Autodesk Inventor part; units mm, degrees
ref_plane "YZ Plane" through (0, 0, 0) normal (1, 0, 0) x (0, 1, 0)
ref_plane "XZ Plane" through (0, 0, 0) normal (0, 1, 0) x (-1, 0, 0)
ref_plane "XY Plane" through (0, 0, 0) normal (0, 0, 1) x (1, 0, 0)
sketch "Sketch1" plane through (0, 0, 0) normal (1, 0, 0) x (0, 1, 0)
  line L0 (0, 0) -> (103.378, 0)
  line L1 (103.378, 0) -> (103.378, -444.5)
  line L2 (103.378, -444.5) -> (0, -444.5)
  line L3 (0, -444.5) -> (0, 0)
  circle A0 centre (31.75, -50.8) radius 6.3627
  circle A1 centre (31.75, -393.7) radius 6.3627
  circle A2 centre (88.0618, -165.5318) radius 1.5875
  circle A3 centre (72.0598, -165.5318) radius 1.5875
  circle A4 centre (15.3162, -278.9682) radius 1.5875
  circle A5 centre (31.3182, -278.9682) radius 1.5875
  dimension "d0" = 103.378
  dimension "d1" = 444.5
  dimension "d2" = 12.7254
  dimension "d3" = 31.75
  dimension "d4" = 50.8
  dimension "d5" = 50.8
  dimension "d22" = 165.5318
  dimension "d23" = 3.175
  dimension "d24" = 15.3162
  dimension "d25" = 3.175
  dimension "d26" = 16.002
  dimension "d27" = 165.5318
  dimension "d28" = 3.175
  dimension "d29" = 15.3162
  dimension "d30" = 165.5318
  dimension "d31" = 3.175
  dimension "d32" = 16.002
  dimension "d33" = 165.5318
extrude "Extrusion1" add sketch "Sketch1" along normal blind 6.35 contours L0 L1 L2 L3 | A2 | A3 | A4 | A5
chamfer "Chamfer1" distance 38.1 angle 45 1 edges at (3.175, 0, 0)
chamfer "Chamfer2" distance 38.1 angle 45 1 edges at (3.175, 0, -444.5)
sketch "Sketch2" plane through (6.35, 0, 0) normal (1, 0, 0) x (0, 0, -1)
  line L0 (444.5, 38.1) -> (406.4, 0)
  line L1 (444.5, 38.1) -> (444.5, 103.378)
  line L2 (444.5, 103.378) -> (0, 103.378)
  line L3 (0, 103.378) -> (0, 38.1)
  line L4 (38.1, 0) -> (0, 38.1)
  line L5 (38.1, 0) -> (406.4, 0)
  circle A0 centre (393.7, 31.75) radius 6.3627
  circle A1 centre (50.8, 31.75) radius 6.3627
  circle A2 centre (120.4214, 66.0654) radius 6.3627
  circle A3 centre (324.0786, 37.3126) radius 6.3627
  point P0 (0, 0)
  dimension "d14" = 12.7254
  dimension "d15" = 120.4214
  dimension "d16" = 37.3126
  dimension "d17" = 12.7254
  dimension "d18" = 37.3126
  dimension "d19" = 120.4214
extrude "Extrusion2" cut sketch "Sketch2" against normal blind 25.4 contours A2 | A3
sketch "Sketch3" plane through (6.35, 0, 0) normal (1, 0, 0) x (0, 0, -1)
  circle A0 centre (120.4214, 66.0654) radius 6.3627
  circle A1 centre (324.0786, 37.3126) radius 6.3627
  line L0 (444.5, 38.1) -> (406.4, 0)
  line L1 (444.5, 38.1) -> (444.5, 103.378)
  line L2 (444.5, 103.378) -> (0, 103.378)
  line L3 (0, 103.378) -> (0, 38.1)
  line L4 (38.1, 0) -> (0, 38.1)
  line L5 (38.1, 0) -> (406.4, 0)
  circle A2 centre (393.7, 31.75) radius 6.3627
  circle A3 centre (50.8, 31.75) radius 6.3627
  circle A4 centre (165.5318, 88.0618) radius 1.5875
  circle A5 centre (165.5318, 72.0598) radius 1.5875
  circle A6 centre (278.9682, 15.3162) radius 1.5875
  circle A7 centre (278.9682, 31.3182) radius 1.5875
  point P0 (0, 0)
  dimension "d34" = 3.175
  dimension "d35" = 165.5318
  dimension "d36" = 15.3162
  dimension "d37" = 3.175
  dimension "d38" = 16.002
  dimension "d39" = 3.175
  dimension "d40" = 3.175
  dimension "d41" = 15.3162
  dimension "d42" = 16.002
  dimension "d43" = 165.5318
extrude "Extrusion3" cut sketch "Sketch3" against normal blind 25.4 contours A4 | A5 | A6 | A7
sketch "Sketch4" plane through (6.35, 0, 0) normal (1, 0, 0) x (0, 0, -1)
  circle A0 centre (278.9682, 15.3162) radius 1.5875
  circle A1 centre (165.5318, 88.0618) radius 1.5875
  circle A2 centre (165.5318, 72.0598) radius 1.5875
  circle A3 centre (278.9682, 31.3182) radius 1.5875
  circle A4 centre (120.4214, 66.0654) radius 6.3627
  circle A5 centre (324.0786, 37.3126) radius 6.3627
  line L0 (444.5, 38.1) -> (406.4, 0)
  line L1 (444.5, 38.1) -> (444.5, 103.378)
  line L2 (444.5, 103.378) -> (0, 103.378)
  line L3 (0, 103.378) -> (0, 38.1)
  line L4 (38.1, 0) -> (0, 38.1)
  line L5 (38.1, 0) -> (406.4, 0)
  circle A6 centre (393.7, 31.75) radius 6.3627
  circle A7 centre (50.8, 31.75) radius 6.3627
  arc A8 (50.165, 90.3605) -> (50.165, 80.8355) centre (50.165, 85.598) ccw
  arc A9 (67.31, 80.8355) -> (67.31, 90.3605) centre (67.31, 85.598) ccw
  line L6 (50.165, 80.8355) -> (67.31, 80.8355)
  line L7 (67.31, 90.3605) -> (50.165, 90.3605)
  arc A10 (393.5026, 80.9088) -> (394.4579, 90.3589) centre (394.335, 85.598) ccw
  arc A11 (375.9516, 90.3589) -> (376.3576, 80.9088) centre (376.7145, 85.6579) ccw
  line L8 (376.3576, 80.9088) -> (393.5026, 80.9088)
  line L9 (394.4579, 90.3589) -> (375.9516, 90.3589)
  point P0 (0, 0)
  dimension "d46" = 9.525
  dimension "d47" = 50.165
  dimension "d48" = 17.78
  dimension "d49" = 9.525
  dimension "d50" = 17.145
  dimension "d51" = 9.525
  dimension "d52" = 50.165
  dimension "d53" = 17.78
  dimension "d54" = 9.525
  dimension "d56" = 17.145
extrude "Extrusion4" cut sketch "Sketch4" against normal blind 25.4 contours L7 A9 L6 A8 | L8 A11 L9 A10
sketch "Sketch5" plane through (6.35, 0, 0) normal (1, 0, 0) x (0, 0, -1)
  line L0 (67.31, 80.8355) -> (50.165, 80.8355)
  arc A0 (50.165, 90.3605) -> (50.165, 80.8355) centre (50.165, 85.598) ccw
  line L1 (50.165, 90.3605) -> (67.31, 90.3605)
  arc A1 (67.31, 80.8355) -> (67.31, 90.3605) centre (67.31, 85.598) ccw
  line L2 (393.5026, 80.9088) -> (376.3576, 80.9088)
  arc A2 (375.9516, 90.3589) -> (376.3576, 80.9088) centre (376.7145, 85.6579) ccw
  line L3 (375.9516, 90.3589) -> (394.4579, 90.3589)
  arc A3 (393.5026, 80.9088) -> (394.4579, 90.3589) centre (394.335, 85.598) ccw
  circle A4 centre (278.9682, 15.3162) radius 1.5875
  circle A5 centre (165.5318, 88.0618) radius 1.5875
  circle A6 centre (165.5318, 72.0598) radius 1.5875
  circle A7 centre (278.9682, 31.3182) radius 1.5875
  circle A8 centre (120.4214, 66.0654) radius 6.3627
  circle A9 centre (324.0786, 37.3126) radius 6.3627
  line L4 (444.5, 38.1) -> (406.4, 0)
  line L5 (444.5, 38.1) -> (444.5, 103.378)
  line L6 (444.5, 103.378) -> (0, 103.378)
  line L7 (0, 103.378) -> (0, 38.1)
  line L8 (38.1, 0) -> (0, 38.1)
  line L9 (38.1, 0) -> (406.4, 0)
  circle A10 centre (393.7, 31.75) radius 6.3627
  circle A11 centre (50.8, 31.75) radius 6.3627
  circle A12 centre (16.51, 98.298) radius 2.159
  circle A13 centre (16.51, 72.898) radius 2.159
  circle A14 centre (427.99, 98.298) radius 2.159
  circle A15 centre (427.99, 72.898) radius 2.159
  point P0 (0, 0)
  dimension "d59" = 4.318
  dimension "d60" = 16.51
  dimension "d61" = 5.08
  dimension "d62" = 4.318
  dimension "d63" = 25.4
  dimension "d64" = 4.318
  dimension "d65" = 4.318
  dimension "d66" = 5.08
  dimension "d67" = 25.4
  dimension "d68" = 16.51
extrude "Extrusion5" cut sketch "Sketch5" against normal blind 25.4 contours A12 | A13 | A14 | A15
properties part number "DriveTrain3.0"
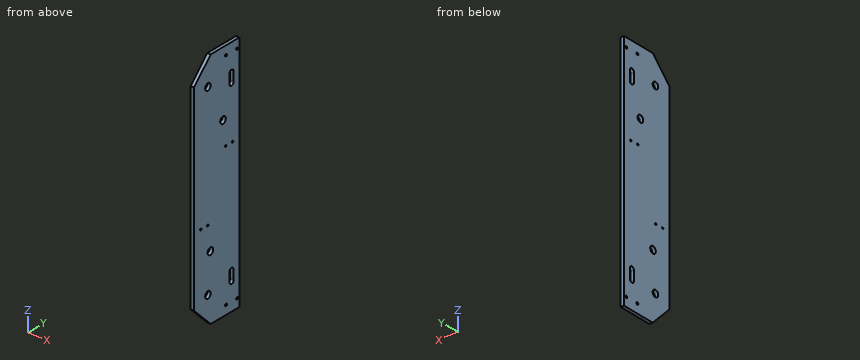
CAD build for the part. Positions are in the model's coordinates, mm. Round coordinates to 2 decimals unless told otherwise and drop trailing zeros. Order: outer loops, then holes, each group sorted by start corner. A loop starts at its lowest first (then second) coordinate and runs counter-clockwise, first axis right, second up. Notation, with made-up numbers: (-32, -36) -> (13, -36) arc R27 ccw to (13, -18) -> close; hole circle Ø2 at (65.25, 24). An arc over 180 degrees is marked (long way). Write each question's results on one line, items separated by ' | '.
1. Wall check: line 1 along Y through (x, z) = (5.25, -393.7); line 2 along Y through (x, z) = (2.25, -48.5); line 3 along Z through (x, y) = (4.5, 31.75). Give the ranges that are in metal, low to high. Write a range as [from, to].
Findings below:
line 1: y = [0, 25.39], [38.11, 80.88], [90.36, 103.38] | line 2: y = [0, 25.82], [37.68, 81.14], [90.06, 103.38] | line 3: z = [-438.15, -400.06], [-387.34, -327.17], [-320.99, -280.5], [-277.44, -57.16], [-44.44, -6.35]
2. Cut at B-B (z = -26.5). Give the cut face in (x, y).
Findings below:
outline: (0, 11.6) -> (6.35, 11.6) -> (6.35, 103.38) -> (0, 103.38) -> close
3. Cut at A-A (x = 4.5). Count the separate pieces of the cut face and the enclosed holes in it, plus the area to 3 significant figures.
Findings below:
separate pieces: 1 | enclosed holes: 14 | area: 43,400 mm²
